Autodesk Inventor part; units mm, degrees
ref_plane "YZ Plane" through (0, 0, 0) normal (1, 0, 0) x (0, 1, 0)
ref_plane "XZ Plane" through (0, 0, 0) normal (0, 1, 0) x (-1, 0, 0)
ref_plane "XY Plane" through (0, 0, 0) normal (0, 0, 1) x (1, 0, 0)
sketch "Эскиз1" plane through (0, 0, 0) normal (0, 0, 1) x (1, 0, 0)
  line L0 (-16, -10) -> (34, -10)
  line L1 (38, -6) -> (38, 16)
  line L2 (34, 20) -> (-16, 20)
  line L3 (-20, 16) -> (-20, -6)
  line L4 (-20, 16) -> (-16, 20)
  line L5 (-16, -10) -> (-20, -6)
  line L6 (34, 20) -> (38, 16)
  line L7 (34, -10) -> (38, -6)
  line L8 (-18, -13.8) -> (-18, 33.1) construction
  line L9 (36, -15.5) -> (36, 27.4) construction
  line L10 (-22.5, 15) -> (39.4, 15) construction
  line L11 (-26.6, 10) -> (40.2, 10) construction
  line L12 (-27.2, 5) -> (41.5, 5) construction
  line L13 (-27.8, 0) -> (41.6, 0) construction
  line L14 (-27.6, -5) -> (40.5, -5) construction
  line L15 (-17.5, -12) -> (35.5, -12)
  line L16 (39.5, -8) -> (39.5, 18)
  line L17 (35.5, 22) -> (-17.5, 22)
  line L18 (-21.5, 18) -> (-21.5, -8)
  line L19 (-21.5, 18) -> (-17.5, 22)
  line L20 (39.5, -8) -> (35.5, -12)
  line L21 (39.5, 18) -> (35.5, 22)
  line L22 (39.5, -8) -> (35.5, -12)
  line L23 (-21.5, -8) -> (-17.5, -12)
  point P0 (-20, -10)
  point P1 (38, 20)
  point P2 (38, -10)
  point P3 (-20, 20)
  point P4 (-18, 15)
  point P5 (-18, 10)
  point P6 (-18, 5)
  point P7 (36, 15)
  point P8 (36, 10)
  point P9 (36, 5)
  point P10 (36, 0)
  point P11 (36, -5)
  point P12 (-21.5, -12)
  point P13 (39.5, 22)
  point P14 (39.5, -12)
  point P15 (-21.5, 22)
  point P16 (39.5, -12)
  dimension "d0" = 58
  dimension "d1" = 30
  dimension "d2" = 4
  dimension "d3" = 4
  dimension "d4" = 4
  dimension "d5" = 4
  dimension "d6" = 4
  dimension "d7" = 4
  dimension "d8" = 4
  dimension "d9" = 4
  dimension "d12" = 2
  dimension "d13" = 2
  dimension "d14" = 5
  dimension "d15" = 5
  dimension "d16" = 5
  dimension "d17" = 5
  dimension "d18" = 5
  dimension "d42" = 2
  dimension "d43" = 2
  dimension "d44" = 1.5
  dimension "d45" = 1.5
  dimension "d46" = 4
  dimension "d47" = 4
  dimension "d48" = 4
  dimension "d49" = 4
  dimension "d50" = 4
  dimension "d51" = 4
  dimension "d52" = 4
  dimension "d53" = 4
  dimension "d54" = 4
  dimension "d55" = 4
extrude "Выдавливание2" add sketch "Эскиз1" along normal blind 2
equation "\"Радиус_гибки\" = Толщина"
equation "\"Ширина_просечки\" = Толщина"
equation "\"Глубина_просечки\" = 0.5 * Толщина"
equation "\"Размер_высечки\" = 4 * Толщина"
equation "\"Мин_остаток\" = 2 * Толщина"
equation "\"Радиус_перехода\" = Радиус_гибки"
equation "\"Радиус_Якоби\" = Радиус_гибки"
equation "\"Размер_зазора\" = Толщина"
properties part number "клей" material "По умолчанию"
Can you work these out from the model? Positions are in its coordinate system, mm. A direction names the side the tool comes from. Coordinates: 2 decimals unless noted, no trailing zeros. Loops run counter-clockwise (first coordinate to the right, second up) from the corner with the lowest first, then second, coordinate; pieces in that order, holes last. Notation, with made-up numbers: (22, 55.5) - (38, 55.5) arc R23 ccw to (38, 85.5) - close; hole circle Ø8 at (-21, -34.5). An arc over 180 degrees is marked (long way). Answer as a JSON object with one key per item and string values. Group by question number.
Item 1: If I drill on L1, parallel to X at y = 8, z = 0.45; L2, parallel to Y at x = 14.5, z = 0.4; L3, parallel to X at y = 18.5, z = 1.2, over which ranges is the centre line in solid material (lowest first)? Write a range as from..to.
Item 2: If we section it at B-B (x = -7.5): List the corners of the cut face in (y, z) for me, plus the area to 3 significant figures.
Item 3: On a 3-axis mill with a long thin cutter (end or side, diameter ignored), from which of +Z, -Z, +X, -X, +Y, -Y can I reach the whole of each face in a straight line? I mean faces 5 (the face through (-18, 18, 1)), 6 (the face through (-19.5, 20, 1)). Say none if no direction works.
Item 4: If we section it at A-A (y = 17): List the corners of the cut face in (x, z) for me, plus the area to 3 significant figures.
Item 5: If we mould it in two halves opening along Y, with no side actions, what happens to faces 1 (the face through (37.5, -10, 1)), 2 (the face through (-21.5, 5, 1)), 3 (the face through (-20, 5, 1)), 4 (the face through (36, 18, 1))? For each: released by +Y, released by -Y, zero draft, split by the parting line, or undercut.
Item 6: If we section it at C-C (z = 1.2): List the corners of the cut face in (x, y) for me.
Returned:
{
 "1": {"L1": "x = -21.5..-20, 38..39.5", "L2": "y = -12..-10, 20..22", "L3": "x = -21..-17.5, 35.5..39"},
 "2": {"outline": "(-12, 0) - (-10, 0) - (-10, 2) - (-12, 2) - close; (20, 0) - (22, 0) - (22, 2) - (20, 2) - close", "area": "8.00 mm²"},
 "3": {"face 5": "+Z, -Z", "face 6": "+Z, -Z, -X, +Y"},
 "4": {"outline": "(-21.5, 0) - (-19, 0) - (-19, 2) - (-21.5, 2) - close; (37, 0) - (39.5, 0) - (39.5, 2) - (37, 2) - close", "area": "10.0 mm²"},
 "5": {"face 1": "released by -Y", "face 2": "zero draft", "face 3": "undercut", "face 4": "undercut"},
 "6": {"outline": "(-21.5, -8) - (-17.5, -12) - (35.5, -12) - (39.5, -8) - (39.5, 18) - (35.5, 22) - (-17.5, 22) - (-21.5, 18) - close; hole (-20, -6) - (-16, -10) - (34, -10) - (38, -6) - (38, 16) - (34, 20) - (-16, 20) - (-20, 16) - close"}
}
